Geometry: final body of the model. Coordinates: model frame, mm. A direction names the side the tool comes from. Round coordinates to 2 decimals unless told otherwise and drop trailing zeros. Loops run counter-clockwise (first coordinate to the right, second up) from the corner with the lowest first, then second, coordinate; pieces in that order, holes last. Notation, with made-up numbers: (27, -24.75) - (42, -24.75) arc R17 ccw to (42, -6.75) - close; hole circle Ø11 at (-24, 3.5). An arc over 180 degrees is marked (long way). Write item = value, one per line. Start each with the question number.
Item 1: Draft query along Z for faces 1 (the flat face through (-6, 0, 6)), 2 (the cylindrical face through (-10, -29.6, -3.2)), 3 (the flat face through (-2, -5, 5)). Return one class per face: pulls with the +Z half, pulls with the -Z half, needs draft (parallel to the pull), parting line crosses it, or undercut.
Item 2: Access query for faces 4 (the flat face through (6, -60, 6)), 5 (the cylindrical face through (-12.932, -58.732, 5.362)), 6 (the flat face through (2, -55, 5)), 7 (the cylindrical face through (-4.032, -2.535, -6.324)), 8 (the flat face through (0, -3, 11)). Directions: +Z, -Z, +X, -X, +Y, -Y. A direction counts if a zero-diameter tool reaches every point of the face in a straight line with its end or side. Return the directions, or none.
Item 3: Section B-B (z = 0). Return loops of the section in (x, y).
Item 4: First-contact query: pin 1 (13.5 mm diameter, centred on x = 3.5, z = -4.5, fed in from -Y); pin 2 (9 mm diameter, centred on x = 0, z = 0, fed in from -Y); pin 3 (7.5 mm diameter, centred on x = 2, z = 1, fed in from -Y); pin 4 (4.5 mm diameter, centred on x = -3, z = 2.5, fed in from +Y). Flat tips, straight axial feed; report the tip coordinate or a pass-through.
Item 5: Section C-C (y = -41). Return loops of the section in (x, z).
Item 6: Line query: line 1 (Z direction, x = -0.25, y = -52); line 2 (Y direction, x = 7.5, z = -7.75); line 3 (Z direction, x = -3, y = -23). Output: solid intervals per line, ascending. Write a range as from..to.
Item 7: Section A-A (x = 0). Return loops of the section in (y, z).
from build123d import *

# Parameters (mm, degrees)
CHAMFER_1_SIZE = 0.5


with BuildPart() as part:
    # 草图1 → 旋转1 (revolve)
    with BuildSketch(Plane.XY, mode=Mode.PRIVATE) as revolve_1_sk:
        Polygon((7.5, -55), (7.5, -60), (14, -60), (14, -57), (10.5, -57), (10.5, -3), (14, -3), (14, 0), (7.5, 0), (7.5, -5), (5, -5), (5, -55), align=None)
    revolve(revolve_1_sk.sketch.rotate(Axis((0, 0, 0), (0, -1, 0)), 180), axis=Axis((0, 0, 0), (0, -1, 0)))

    # 倒角1
    chamfer_1_edges = [part.edges().sort_by_distance(p)[0] for p in [
        (14, -3, 0),
        (14, -57, 0),
    ]]
    chamfer(chamfer_1_edges, length=CHAMFER_1_SIZE)


solid = part.part
Taken from the geometry:
q1.face_1 = needs draft
q1.face_2 = parting line crosses it
q1.face_3 = undercut
q2.face_4 = +Z, -Z, +X, -X, -Y
q2.face_5 = +Y, -Y
q2.face_6 = -Y
q2.face_7 = +Y
q2.face_8 = none
q3.outline = (-14, -60) - (-7.5, -60) - (-7.5, -55) - (-5, -55) - (-5, -5) - (-7.5, -5) - (-7.5, 0) - (-14, 0) - (-14, -2.5) - (-13.5, -3) - (-10.5, -3) - (-10.5, -57) - (-13.5, -57) - (-14, -57.5) - close; (5, -55) - (7.5, -55) - (7.5, -60) - (14, -60) - (14, -57.5) - (13.5, -57) - (10.5, -57) - (10.5, -3) - (13.5, -3) - (14, -2.5) - (14, 0) - (7.5, 0) - (7.5, -5) - (5, -5) - close
q4.pin_1 = -60
q4.pin_2 = through
q4.pin_3 = -55
q4.pin_4 = -5
q5.outline = circle Ø21 at (0, 0); hole circle Ø10 at (0, 0)
q6.line_1 = -10.5..-4.99, 4.99..10.5
q6.line_2 = -60..-57, -3..0
q6.line_3 = -10.06..-4, 4..10.06
q7.outline = (-60, -14) - (-57.5, -14) - (-57, -13.5) - (-57, -10.5) - (-3, -10.5) - (-3, -13.5) - (-2.5, -14) - (0, -14) - (0, -7.5) - (-5, -7.5) - (-5, -5) - (-55, -5) - (-55, -7.5) - (-60, -7.5) - close; (-60, 7.5) - (-55, 7.5) - (-55, 5) - (-5, 5) - (-5, 7.5) - (0, 7.5) - (0, 14) - (-2.5, 14) - (-3, 13.5) - (-3, 10.5) - (-57, 10.5) - (-57, 13.5) - (-57.5, 14) - (-60, 14) - close
